For this review, take the finished solid that the model builds, in its own axes (mm). Face numbers are marked on the shaded views. A direction names the side the tool comes from. Round coordinates to 2 decimals unless told otherwise and drop trailing zeros. Loops run counter-clockwise (first coordinate to the right, second up) from the corner with the lowest first, then second, coordinate; pieces in that order, holes last. Notation, with made-up numbers: M 21.25,-9.5 L 62.25,-9.5 A12 cw 62.25,6.5 Z; hole C -9.75,89 d8. An arc over 180 degrees is marked long. One line per question, with ' | ' between items. Start each with the question number.
1) We need section C-C (x = -74). Give the boundary of the cut face in (y, z).
2) We need section D-D (y = -29). Give the boundary of the cut face in (x, z).
3) Mouldability with a two-part tool opening along X and no side actions: class the marked faces 1, 2 and 3 as pulls with the +X half, pulls with the -X half, needs draft (parallel to the pull), parting line crosses it, or undercut.
4) We need section A-A (x = -68). Give the boundary of the cut face in (y, z).
5) We need section B-B (z = 33). Give the boundary of the cut face in (x, y).
6) For pin 1 Ø5 at (y, z) = (-46.5, 32.5) entering from -X; pin 2 Ø17.5 at (y, z) = (-17, -16) entering from -X; pin 3 Ø7.5 at (x, y) = (-68, -34.5) entering from +Z; pin 4 Ø6 at (y, z) = (-45, 33) entering from +X, all flat-tipped, find the tip position at first contact; note any pin that passes through.
7) For probe 1 along Z at (x, y) = (-41, -10); probe 2 along Z at (x, y) = (-72.5, -16.5); probe 3 along Y at (x, z) = (-55, 33.5), list the stretches that pass through material, from the lowest coordinate up. Write a range as from..to.
8) For the marked faces 4, 5 and 6, list the 3-axis set-ups (+Z, -Z, +X, -X, +Y, -Y) from which the entire face can be reached by the end or side of a thin tool; tool diameter is ignored.
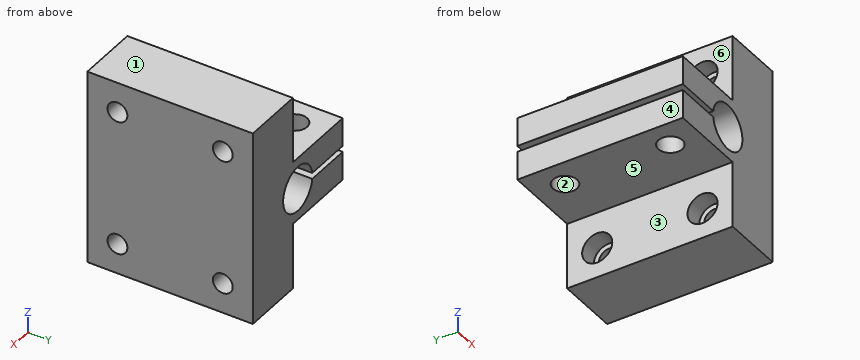
```python
from build123d import *

# Parameters (mm, degrees)
F1_DEPTH = 55
F2_R     = 4
F3_DEPTH = 25
F4_R     = 5
F4_R_2   = 3.3
F5_DEPTH = 6
F6_DEPTH = 25
F7_R     = 5
F7_R_2   = 3.3
F8_DEPTH = 6
F9_DEPTH = 25


with BuildPart() as f1:
    # F0 (on Front) → F1 (new body)
    with BuildSketch(Plane.XZ):
        with BuildLine():
            Line((-36.317323, 43), (-56.817323, 43))
            Line((-56.817323, 43), (-56.817323, 21))
            Line((-56.817323, 21), (-82.317323, 21))
            Line((-82.317323, 21), (-82.317323, 11.5))
            Line((-82.317323, 11.5), (-66.750358, 11.5))
            ThreePointArc((-66.750358, 11.5), (-51.817323, 10.5), (-66.750358, 9.5))
            Line((-66.750358, 9.5), (-82.317323, 9.5))
            Line((-82.317323, 9.5), (-82.317323, 0))
            Line((-82.317323, 0), (-56.817323, 0))
            Line((-56.817323, 0), (-56.817323, -22))
            Line((-56.817323, -22), (-36.317323, -22))
            Line((-36.317323, -22), (-36.317323, 43))
        make_face()
    extrude(amount=F1_DEPTH)

    # F2 (on face) → F3 (cut)
    with BuildSketch(Plane.XY.offset(21)):
        with Locations((-73.317323, -10)):
            Circle(F2_R)
        with Locations((-73.317323, -45)):
            Circle(F2_R)
    extrude(amount=-F3_DEPTH, mode=Mode.SUBTRACT)

    # F4 (on face) → F5 (cut)
    with BuildSketch(Plane(origin=(-56.817323, 0, 0), x_dir=(0, -1, 0), z_dir=(-1, 0, 0))):
        with Locations((10, -12)):
            Circle(F4_R)
        with Locations((10, -12)):
            Circle(F4_R_2, mode=Mode.SUBTRACT)
        with Locations((10, -12)):
            Circle(F4_R_2)
        with Locations((45, -12)):
            Circle(F4_R_2)
        with Locations((45, -12)):
            Circle(F4_R)
        with Locations((45, -12)):
            Circle(F4_R_2, mode=Mode.SUBTRACT)
    extrude(amount=-F5_DEPTH, mode=Mode.SUBTRACT)

    # F4 (on face) → F6 (cut)
    with BuildSketch(Plane(origin=(-56.817323, 0, 0), x_dir=(0, -1, 0), z_dir=(-1, 0, 0))):
        with Locations((10, -12)):
            Circle(F4_R_2)
        with Locations((45, -12)):
            Circle(F4_R_2)
    extrude(amount=-F6_DEPTH, mode=Mode.SUBTRACT)

    # F7 (on face) → F8 (cut)
    with BuildSketch(Plane(origin=(-56.817323, 0, 0), x_dir=(0, -1, 0), z_dir=(-1, 0, 0))):
        with Locations((10, 33)):
            Circle(F7_R)
        with Locations((10, 33)):
            Circle(F7_R_2, mode=Mode.SUBTRACT)
        with Locations((45, 33)):
            Circle(F7_R)
        with Locations((45, 33)):
            Circle(F7_R_2, mode=Mode.SUBTRACT)
    extrude(amount=-F8_DEPTH, mode=Mode.SUBTRACT)

    # F7 (on face) → F9 (cut)
    with BuildSketch(Plane(origin=(-56.817323, 0, 0), x_dir=(0, -1, 0), z_dir=(-1, 0, 0))):
        with Locations((10, 33)):
            Circle(F7_R_2)
        with Locations((45, 33)):
            Circle(F7_R_2)
    extrude(amount=-F9_DEPTH, mode=Mode.SUBTRACT)


solid = f1.part
```
Answers below:
1) outline: M -55,0 L -48.94,0 L -48.94,9.5 L -55,9.5 Z; M -55,11.5 L -48.94,11.5 L -48.94,21 L -55,21 Z; M -41.06,0 L -13.94,0 L -13.94,9.5 L -41.06,9.5 Z; M -41.06,11.5 L -13.94,11.5 L -13.94,21 L -41.06,21 Z; M -6.06,0 L 0,0 L 0,9.5 L -6.06,9.5 Z; M -6.06,11.5 L 0,11.5 L 0,21 L -6.06,21 Z
2) outline: M -82.32,0 L -56.82,0 L -56.82,-22 L -36.32,-22 L -36.32,43 L -56.82,43 L -56.82,21 L -82.32,21 L -82.32,11.5 L -66.75,11.5 A7.5 cw long -66.75,9.5 L -82.32,9.5 Z
3) face 1: needs draft | face 2: undercut | face 3: pulls with the -X half
4) outline: M -55,0 L 0,0 L 0,9.5 L -55,9.5 Z; M -55,11.5 L 0,11.5 L 0,21 L -55,21 Z
5) outline: M -56.82,-55 L -36.32,-55 L -36.32,-48.3 L -50.82,-48.3 L -50.82,-50 L -56.82,-50 Z; M -56.82,-40 L -50.82,-40 L -50.82,-41.7 L -36.32,-41.7 L -36.32,-13.3 L -50.82,-13.3 L -50.82,-15 L -56.82,-15 Z; M -56.82,-5 L -50.82,-5 L -50.82,-6.7 L -36.32,-6.7 L -36.32,0 L -56.82,0 Z
6) pin 1: x = -50.82 | pin 2: x = -56.82 | pin 3: z = 21 | pin 4: through
7) probe 1: -22..-15.3, -8.7..29.7, 36.3..43 | probe 2: 0..9.5, 11.5..21 | probe 3: -55..-49.97, -40.03..-14.97, -5.03..0
8) face 4: +Z, -Z, -X, +Y, -Y | face 5: -Z, -X, +Y, -Y | face 6: +Z, -X, +Y, -Y
